For this review, take the finished solid that the model builds, in its own axes (mm). Face numbers are marked on the shaded views. Round coordinates to 2 decimals unless told otherwise and drop trailing zeros. Write each loop counter-clockwise with the first axis right and the second up, starting at its lowest first coordinate (ties: lowest second). Pieces come first, ordered by that corner, then holes. Notation, with made-up numbers: (-7.5, 33.5) -> (0.5, 33.5) arc R9 ccw to (0.5, 43.5) -> close; hole circle Ø3 at (7.25, -27). An arc over 180 degrees is marked (long way). Answer in a Markdown table with one row per item. Add a question column.
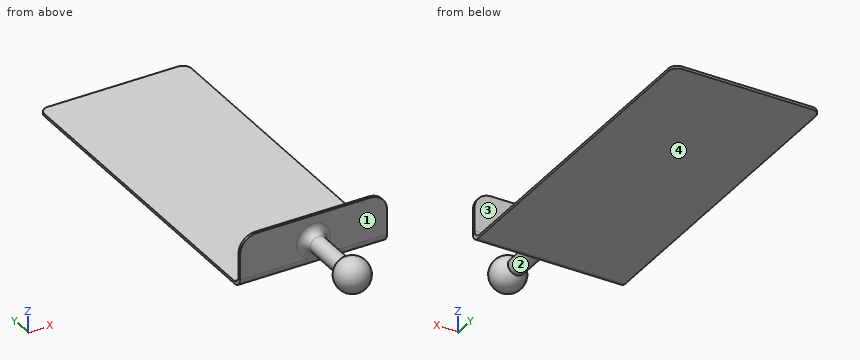
```python
from build123d import *

# Parameters (mm, degrees)
SKETCH1_W           = 87
SKETCH1_H           = 1.5
BOSS_EXTRUDE1_DEPTH = 200
SKETCH2_W           = 87
SKETCH2_H           = 1.5
BOSS_EXTRUDE2_DEPTH = 28.5
FILLET1_R           = 5
FILLET2_R           = 5
FILLET3_R           = 5
FILLET4_R           = 10


with BuildPart() as part:
    # Sketch1 → Boss-Extrude1 (new body)
    with BuildSketch(Plane(origin=(0, 0, 0), x_dir=(1, 0, 0), z_dir=(0, 1, 0))):
        Rectangle(SKETCH1_W, SKETCH1_H)
    extrude(amount=BOSS_EXTRUDE1_DEPTH)

    # Sketch2 → Boss-Extrude2 (add)
    with BuildSketch(Plane.XY.offset(0.75)):
        with Locations((0, 0.75)):
            Rectangle(SKETCH2_W, SKETCH2_H)
    extrude(amount=BOSS_EXTRUDE2_DEPTH)

    # Fillet1
    fillet1_edges = [part.edges().sort_by_distance(p)[0] for p in [
        (0, 1.5, 0.75),
        (0, 0, -0.75),
    ]]
    fillet(fillet1_edges, radius=FILLET1_R)

    # Sketch4 → Revolve1 (revolve)
    with BuildSketch(Plane.XY.offset(14.25), mode=Mode.PRIVATE) as revolve1_sk:
        with BuildLine():
            Line((5, 0), (5, -30))
            ThreePointArc((5, -30), (9.659258263, -41.248444489), (0, -48.660254038))
            Line((0, -48.660254038), (0, 0))
            Line((0, 0), (0, 0.59177988))
            Line((0, 0.59177988), (5, 0.59177988))
            Line((5, 0.59177988), (5, 0))
        make_face()
    revolve(revolve1_sk.sketch.rotate(Axis((0, 0, 14.25), (0, -1, 0)), 180), axis=Axis((0, 0, 14.25), (0, -1, 0)))

    # Fillet2
    fillet2_edges = [part.edges().sort_by_distance(p)[0] for p in [
        (5, 0, 14.25),
    ]]
    fillet(fillet2_edges, radius=FILLET2_R - 0.0001)  # a hair under: the kernel refuses the full size

    # Fillet3
    fillet3_edges = [part.edges().sort_by_distance(p)[0] for p in [
        (43.5, 200, 0),
        (-43.5, 200, 0),
    ]]
    fillet(fillet3_edges, radius=FILLET3_R)

    # Fillet4
    fillet4_edges = [part.edges().sort_by_distance(p)[0] for p in [
        (-43.5, 0.75, 29.25),
        (43.5, 0.75, 29.25),
    ]]
    fillet(fillet4_edges, radius=FILLET4_R)


solid = part.part
```
1. Clearance check with flat-ended pins moving along their axes: pin 1 Ø1.5 at (y, z) = (-16, 15) entering from +X; pin 2 Ø12 at (x, z) = (-20.5, 19) entering from +Y; pin 3 Ø2 at (x, y) = (-23.5, 112.5) entering from +Z. State where each tip first meets the part, or that it passes through.
2. We need section B-B (z = 14.25). Write out the cut boundary in (x, y), plus the area to 3 significant figures.
3. The part is to be moulded in two halves that separate along Y. For the marked faces 1, 2, 3 and 4, say which applies: pulls with the +Y half, pulls with the -Y half, needs draft (parallel to the pull), parting line crosses it, or undercut.
4. We need section C-C (x = 30.5). Write out the cut boundary in (y, z), plus the area to 3 significant figures.
5. For L1, parallel to Y at x = -36, z = 27.75; L2, parallel to Z at x = 9, y = 114.5, list the stretches that pass through material, from the lowest coordinate up. Write a range as [from, to].
6. We need section D-D (y = 110). Write out the cut boundary in (x, z), plus the area to 4 significant figures.
Response:
| question | item | result |
|---|---|---|
| 1 | pin 1 | x = 5 |
| 1 | pin 2 | y = 1.5 |
| 1 | pin 3 | z = 0.75 |
| 2 | outline | (-43.5, 0) -> (-10, 0) arc R5 cw to (-5, -5) -> (-5, -30) arc R10 ccw (long way) to (5, -30) -> (5, -5) arc R5 cw to (10, 0) -> (43.5, 0) -> (43.5, 1.5) -> (-43.5, 1.5) -> close |
| 2 | area | 746 mm2 |
| 3 | face 1 | pulls with the -Y half |
| 3 | face 2 | undercut |
| 3 | face 3 | pulls with the +Y half |
| 3 | face 4 | needs draft |
| 4 | outline | (0, 4.25) arc R5 ccw to (5, -0.75) -> (200, -0.75) -> (200, 0.75) -> (6.5, 0.75) arc R5 cw to (1.5, 5.75) -> (1.5, 29.25) -> (0, 29.25) -> close |
| 4 | area | 343 mm2 |
| 5 | L1 | [0, 1.5] |
| 5 | L2 | [-0.75, 0.75] |
| 6 | outline | (-43.5, -0.75) -> (43.5, -0.75) -> (43.5, 0.75) -> (-43.5, 0.75) -> close |
| 6 | area | 130.5 mm2 |
